Can you work these out from the model? Positions are in its coordinate system, mm. A direction names the side the tool comes from. Coordinates: 2 decimals unless noted, no trailing zeros. Order: outer loops, then holes, each group sorted by start corner. A loop starts at its lowest first (then second) coordinate and runs counter-clockwise, first axis right, second up.
```python
from build123d import *

# Parameters (mm, degrees)
BOSS_EXTRUDE1_DEPTH = 6
SKETCH1_7_R         = 2.5
SKETCH1_7_R_2       = 3.6
SKETCH1_7_R_3       = 15
CUT_EXTRUDE3_DEPTH  = 6


with BuildPart() as part:
    # Sketch1 → Boss-Extrude1 (new body)
    with BuildSketch(Plane(origin=(0, 0, 0), x_dir=(1, 0, 0), z_dir=(0, 1, 0))):
        Polygon((39.199236391, -39.199236391), (39.199236391, 39.199236391), (-75.800763609, 39.199236391), (-75.800763609, -39.199236391), (-39.199236391, -39.199236391), align=None)
    extrude(amount=BOSS_EXTRUDE1_DEPTH)

    # Sketch1<7> → Cut-Extrude3 (cut)
    with BuildSketch(Plane(origin=(0, 0, 0), x_dir=(1, 0, 0), z_dir=(0, 1, 0))):
        with Locations((-18.568778226, 29.199236391)):
            Circle(SKETCH1_7_R)
        with Locations((-18.568778226, -14.199236391)):
            Circle(SKETCH1_7_R)
        with Locations((24.199236391, 29.199236391)):
            Circle(SKETCH1_7_R)
        with Locations((9.199236391, 29.199236391)):
            Circle(SKETCH1_7_R)
        with Locations((21.131221774, 0)):
            Circle(SKETCH1_7_R_2)
        Circle(SKETCH1_7_R)
        with Locations((-10, 0)):
            Circle(SKETCH1_7_R)
        with Locations((-18.568778226, 0)):
            Circle(SKETCH1_7_R)
        with Locations((10, 0)):
            Circle(SKETCH1_7_R)
        with Locations((-5.800763609, 29.199236391)):
            Circle(SKETCH1_7_R)
        with Locations((-5.800763609, -29.199236391)):
            Circle(SKETCH1_7_R)
        with Locations((24.199236391, -29.199236391)):
            Circle(SKETCH1_7_R)
        with Locations((9.199236391, -29.199236391)):
            Circle(SKETCH1_7_R)
        with Locations((0, -9.199236391)):
            Circle(SKETCH1_7_R)
        with Locations((0, 10.800763609)):
            Circle(SKETCH1_7_R)
        with Locations((-50, 0)):
            Circle(SKETCH1_7_R_3)
        with BuildLine():
            Line((-68.5, 14), (-62.5, 14))
            ThreePointArc((-62.5, 14), (-61, 15.5), (-62.5, 17))
            Line((-62.5, 17), (-68.5, 17))
            ThreePointArc((-68.5, 17), (-70, 15.5), (-68.5, 14))
        make_face()
        with BuildLine():
            Line((-37.5, 14), (-31.5, 14))
            ThreePointArc((-31.5, 14), (-30, 15.5), (-31.5, 17))
            Line((-31.5, 17), (-37.5, 17))
            ThreePointArc((-37.5, 17), (-39, 15.5), (-37.5, 14))
        make_face()
        with BuildLine():
            Line((-37.5, -17), (-31.5, -17))
            ThreePointArc((-31.5, -17), (-30, -15.5), (-31.5, -14))
            Line((-31.5, -14), (-37.5, -14))
            ThreePointArc((-37.5, -14), (-39, -15.5), (-37.5, -17))
        make_face()
        with BuildLine():
            Line((-68.5, -17), (-62.5, -17))
            ThreePointArc((-62.5, -17), (-61, -15.5), (-62.5, -14))
            Line((-62.5, -14), (-68.5, -14))
            ThreePointArc((-68.5, -14), (-70, -15.5), (-68.5, -17))
        make_face()
    extrude(amount=CUT_EXTRUDE3_DEPTH, mode=Mode.SUBTRACT)


solid = part.part
```
1. Imagine slicing it at C-C on x = -51. Please give me the cut outline in (y, z), then the cut area to 3 significant figures.
Completed:
outline: (0, -39.2) - (6, -39.2) - (6, -14.97) - (0, -14.97) - close; (0, 14.97) - (6, 14.97) - (6, 39.2) - (0, 39.2) - close
area: 291 mm2
2. Imagine slicing it at A-A on x = 0. Please give me the cut outline in (y, z), then the cut area to 3 significant figures.
Completed:
outline: (0, -39.2) - (6, -39.2) - (6, -13.3) - (0, -13.3) - close; (0, -8.3) - (6, -8.3) - (6, -2.5) - (0, -2.5) - close; (0, 2.5) - (6, 2.5) - (6, 6.7) - (0, 6.7) - close; (0, 11.7) - (6, 11.7) - (6, 39.2) - (0, 39.2) - close
area: 380 mm2
3. Thinking about a two-plate mould opening in X: for faces 1 (the flat face through (-75.801, 3, -1)), 2 (the cylindrical face through (-17.225, 2.958, -31.307)), 3 (the flat face through (-19, 3, 39.199)), which applies, pulls with the +X half, pulls with the -X half, needs draft (parallel to the pull), parting line crosses it, or undercut?
Completed:
face 1: pulls with the -X half
face 2: undercut
face 3: needs draft
4. I'm going to push a flat-ended pin straight in: pin 1 (3 mm diameter, centred on x = -12, z = -28, fed in from -Y). Where does the tip first touch, or does it pass through?
Completed:
pin 1: stops at y = 0
5. On a 3-axis mill with a long thin cutter (end or side, diameter ignored), from which of +Z, -Z, +X, -X, +Y, -Y can I reach the whole of each face in a straight line? I mean faces 4 (the flat face through (-66, 3, 17)), 5 (the flat face through (-19, 0, -9)). Say none if no direction works.
Completed:
face 4: +Y, -Y
face 5: +Z, -Z, +X, -X, -Y
6. Imagine slicing it at B-B on z = -6.5. Please give me the cut outline in (x, y), then the cut area to 3 significant figures.
Completed:
outline: (-75.8, 0) - (-63.52, 0) - (-63.52, 6) - (-75.8, 6) - close; (-36.48, 0) - (39.2, 0) - (39.2, 6) - (-36.48, 6) - close
area: 528 mm2
7. Imagine slicing it at D-D on y = 4.65. Give the number of separate pieces and of enclosed holes in the cut face, then the cut area to 3 significant figures.
Completed:
separate pieces: 1
enclosed holes: 20
area: 7,890 mm2
8. Please list where these lines run through material, in increasing order: probe 1 along Z at (x, y) = (-37, 4.55); probe 2 along Z at (x, y) = (-68, 1.6); probe 3 along Z at (x, y) = (-50, 2.05).
Completed:
probe 1: z = -39.2 to -17, -14 to -7.48, 7.48 to 14, 17 to 39.2
probe 2: z = -39.2 to -17, -14 to 14, 17 to 39.2
probe 3: z = -39.2 to -15, 15 to 39.2
